Model file for the job. Use its own axes, mm. A direction names the side the tool comes from. Coordinates: 2 decimals unless noted, no trailing zeros. Write each loop counter-clockwise with the first axis right and the second up, starting at its lowest first coordinate (ties: lowest second). Pieces come first, ordered by that corner, then holes. Notation, with made-up numbers: (-11, 0) - (8, 0) arc R25 cw to (8, 27) - close; hole circle Ø10 at (73, 14). An arc over 180 degrees is marked (long way). Put each result on its own line as item: value. Start each with the question number.
1. Saw through at B-B, the plane z = 68. Write the cut outline in (x, y).
2. Pull direction Z, two halves, no side cores. Call faces 3 (the face through (138.4, -12.52, 41.08)), 4 (the face through (7, -25.4, 37)), 5 (the face through (-76.09, -12.52, 7.42)), 6 (the face through (24.914, -13, -1)): released by +Z, released by -Z, zero draft, split by the parting line, or undercut.
3. Saw through at A-A, the plane x = -2.5. Write the cut outline in (y, z).
4. Which spindle directions (+Z, -Z, +X, -X, +Y, -Y) get a long thin tool onto all of the face, cutting with end or side? Do faces 1 (the face through (0.354, -12.522, 20.673)), 2 (the face through (75.2, -12.522, -8.387)). Say none if no direction does.
5. Drill centre lines: L1, parallel to X at y = -13.25, z = 58.5; L2, parallel to X at y = -10.25, z = 65; L3, parallel to X at y = -11, z = 56. Where is each one in solid material? Low to high. Write a range as from..to.
6. Drop flat-ended pins along their axis: P1, Ø4, axis at x = 65, y = -3.5, coming from the +Z side; P2, Ø10, axis at x = -74.5, y = -20.5, coming from the +Z side; P3, Ø4, axis at x = -22.5, y = -6.5, coming from the -Z side. Give the stop position or say it passes through.
7. Saw through at C-C, the plane y = -9.25. Write the cut outline in (x, z), plus the area to 3 significant figures.
8. Saw through at D-D, the plane x = -50.5. Write the cut outline in (y, z), plus the area to 3 significant figures.
```python
from build123d import *

# Parameters (mm, degrees)
F0_R     = 13.5638253362
F1_DEPTH = 25.4
F2_DEPTH = 41.656
F3_DEPTH = 26.162


with BuildPart() as f1:
    # F0 (on Front) → F1 (new body)
    with BuildSketch(Plane.XZ):
        with BuildLine():
            ThreePointArc((42.2479079596, 0), (36.1330221503, -21.892702831), (19.5584797538, -37.4479852152))
            Line((19.5584797538, -37.4479852152), (132.4212052928, 21.4983992089))
            ThreePointArc((132.4212052928, 21.4983992089), (100.6472035915, 41.7404632116), (123.3718206821, 71.7890924196))
            Line((123.3718206821, 71.7890924196), (-99.4221599354, 82.6346792182))
            ThreePointArc((-99.4221599354, 82.6346792182), (-91.712695746, 74.4613506675), (-88.9104630026, 63.580788672))
            ThreePointArc((-88.9104630026, 63.580788672), (-98.9866948233, 44.8085061449), (-120.2003748087, 42.8314324344))
            Line((-120.2003748087, 42.8314324344), (-30.734153315, -28.9878862108))
            ThreePointArc((-30.734153315, -28.9878862108), (-15.5953846777, 39.2641019726), (42.2479079596, 0))
        make_face()
        with BuildLine():
            Line((-30.734153315, -28.9878862108), (-21.6561091574, -36.2753175468))
            ThreePointArc((-21.6561091574, -36.2753175468), (-1.201582142, -42.2308172703), (19.5584797538, -37.4479852152))
            ThreePointArc((19.5584797538, -37.4479852152), (36.1330221503, -21.892702831), (42.2479079596, 0))
            ThreePointArc((42.2479079596, 0), (-15.5953846777, 39.2641019726), (-30.734153315, -28.9878862108))
        make_face()
        with BuildLine():
            ThreePointArc((-19.4369487029, 7.0494087413), (0, 20.6758104674), (19.4369487029, 7.0494087413))
            Line((19.4369487029, 7.0494087413), (24.9135568738, 7.0494087413))
            Line((24.9135568738, 7.0494087413), (24.9135568738, -8.5022896528))
            Line((24.9135568738, -8.5022896528), (18.8467559315, -8.5022896528))
            ThreePointArc((18.8467559315, -8.5022896528), (0, -20.6758104674), (-18.8467559315, -8.5022896528))
            Line((-18.8467559315, -8.5022896528), (-24.5691239834, -8.5022896528))
            Line((-24.5691239834, -8.5022896528), (-24.5691239834, 7.0494087413))
            Line((-24.5691239834, 7.0494087413), (-19.4369487029, 7.0494087413))
        make_face(mode=Mode.SUBTRACT)
        with BuildLine():
            ThreePointArc((123.3718206821, 71.7890924196), (100.6472035915, 41.7404632116), (132.4212052928, 21.4983992089))
            ThreePointArc((132.4212052928, 21.4983992089), (146.1814974644, 30.6406644058), (151.5054987025, 46.2797712983))
            ThreePointArc((151.5054987025, 46.2797712983), (143.0908574497, 65.2681184027), (123.3718206821, 71.7890924196))
        make_face()
        with Locations((125.873775364, 46.2797712983)):
            Circle(F0_R, mode=Mode.SUBTRACT)
        with BuildLine():
            Line((-129.7982639681, 50.536171143), (-120.2003748087, 42.8314324344))
            ThreePointArc((-120.2003748087, 42.8314324344), (-98.9866948233, 44.8085061449), (-88.9104630026, 63.580788672))
            ThreePointArc((-88.9104630026, 63.580788672), (-91.712695746, 74.4613506675), (-99.4221599354, 82.6346792182))
            ThreePointArc((-99.4221599354, 82.6346792182), (-127.7954989327, 79.063190443), (-129.7982639681, 50.536171143))
        make_face()
        with Locations((-111.4352047443, 63.580788672)):
            Circle(F0_R, mode=Mode.SUBTRACT)
        with BuildLine():
            ThreePointArc((18.8467559315, -8.5022896528), (20.2133754238, -4.3484011382), (20.6758104674, 0))
            ThreePointArc((20.6758104674, 0), (20.3637399061, 3.5787198156), (19.4369487029, 7.0494087413))
            Line((19.4369487029, 7.0494087413), (-19.4369487029, 7.0494087413))
            ThreePointArc((-19.4369487029, 7.0494087413), (-20.6609375603, -0.784090309), (-18.8467559315, -8.5022896528))
            Line((-18.8467559315, -8.5022896528), (18.8467559315, -8.5022896528))
        make_face()
        with Locations((-111.4352047443, 63.580788672)):
            Circle(F0_R)
        with Locations((125.873775364, 46.2797712983)):
            Circle(F0_R)
        with BuildLine():
            Line((-19.4369487029, 7.0494087413), (19.4369487029, 7.0494087413))
            ThreePointArc((19.4369487029, 7.0494087413), (0, 20.6758104674), (-19.4369487029, 7.0494087413))
        make_face()
        with BuildLine():
            ThreePointArc((-18.8467559315, -8.5022896528), (0, -20.6758104674), (18.8467559315, -8.5022896528))
            Line((18.8467559315, -8.5022896528), (-18.8467559315, -8.5022896528))
        make_face()
        with BuildLine():
            ThreePointArc((19.4369487029, 7.0494087413), (20.3637399061, 3.5787198156), (20.6758104674, 0))
            ThreePointArc((20.6758104674, 0), (20.2133754238, -4.3484011382), (18.8467559315, -8.5022896528))
            Line((18.8467559315, -8.5022896528), (24.9135568738, -8.5022896528))
            Line((24.9135568738, -8.5022896528), (24.9135568738, 7.0494087413))
            Line((24.9135568738, 7.0494087413), (19.4369487029, 7.0494087413))
        make_face()
        with BuildLine():
            ThreePointArc((-18.8467559315, -8.5022896528), (-20.6609375603, -0.784090309), (-19.4369487029, 7.0494087413))
            Line((-19.4369487029, 7.0494087413), (-24.5691239834, 7.0494087413))
            Line((-24.5691239834, 7.0494087413), (-24.5691239834, -8.5022896528))
            Line((-24.5691239834, -8.5022896528), (-18.8467559315, -8.5022896528))
        make_face()
        with BuildLine():
            ThreePointArc((-129.7982639681, 50.536171143), (-125.5357705386, 46.0155378963), (-120.2003748087, 42.8314324344))
            Line((-120.2003748087, 42.8314324344), (-129.7982639681, 50.536171143))
        make_face()
        with BuildLine():
            ThreePointArc((-30.734153315, -28.9878862108), (-26.4473356759, -32.9457760966), (-21.6561091574, -36.2753175468))
            Line((-21.6561091574, -36.2753175468), (-30.734153315, -28.9878862108))
        make_face()
    extrude(amount=F1_DEPTH)

    # F0 (on Front) → F2 (cut)
    with BuildSketch(Plane.XZ):
        with BuildLine():
            ThreePointArc((-18.8467559315, -8.5022896528), (0, -20.6758104674), (18.8467559315, -8.5022896528))
            Line((18.8467559315, -8.5022896528), (-18.8467559315, -8.5022896528))
        make_face()
        with BuildLine():
            Line((-19.4369487029, 7.0494087413), (19.4369487029, 7.0494087413))
            ThreePointArc((19.4369487029, 7.0494087413), (0, 20.6758104674), (-19.4369487029, 7.0494087413))
        make_face()
        with BuildLine():
            ThreePointArc((-18.8467559315, -8.5022896528), (-20.6609375603, -0.784090309), (-19.4369487029, 7.0494087413))
            Line((-19.4369487029, 7.0494087413), (-24.5691239834, 7.0494087413))
            Line((-24.5691239834, 7.0494087413), (-24.5691239834, -8.5022896528))
            Line((-24.5691239834, -8.5022896528), (-18.8467559315, -8.5022896528))
        make_face()
        with BuildLine():
            ThreePointArc((19.4369487029, 7.0494087413), (20.3637399061, 3.5787198156), (20.6758104674, 0))
            ThreePointArc((20.6758104674, 0), (20.2133754238, -4.3484011382), (18.8467559315, -8.5022896528))
            Line((18.8467559315, -8.5022896528), (24.9135568738, -8.5022896528))
            Line((24.9135568738, -8.5022896528), (24.9135568738, 7.0494087413))
            Line((24.9135568738, 7.0494087413), (19.4369487029, 7.0494087413))
        make_face()
        with BuildLine():
            ThreePointArc((18.8467559315, -8.5022896528), (20.2133754238, -4.3484011382), (20.6758104674, 0))
            ThreePointArc((20.6758104674, 0), (20.3637399061, 3.5787198156), (19.4369487029, 7.0494087413))
            Line((19.4369487029, 7.0494087413), (-19.4369487029, 7.0494087413))
            ThreePointArc((-19.4369487029, 7.0494087413), (-20.6609375603, -0.784090309), (-18.8467559315, -8.5022896528))
            Line((-18.8467559315, -8.5022896528), (18.8467559315, -8.5022896528))
        make_face()
    extrude(amount=F2_DEPTH, mode=Mode.SUBTRACT)

    # F0 (on Front) → F3 (cut)
    with BuildSketch(Plane.XZ):
        with Locations((-111.4352047443, 63.580788672)):
            Circle(F0_R)
        with Locations((125.873775364, 46.2797712983)):
            Circle(F0_R)
    extrude(amount=F3_DEPTH, mode=Mode.SUBTRACT)


solid = f1.part
```
Final values:
1. outline: (-133.52, -25.4) - (-124.26, -25.4) - (-124.26, 0) - (-133.52, 0) - close; (-98.61, -25.4) - (139.48, -25.4) - (139.48, 0) - (-98.61, 0) - close
2. face 3: undercut
2. face 4: zero draft
2. face 5: released by -Z
2. face 6: undercut
3. outline: (-25.4, -42.17) - (0, -42.17) - (0, -20.52) - (-25.4, -20.52) - close; (-25.4, 20.52) - (0, 20.52) - (0, 77.92) - (-25.4, 77.92) - close
4. face 1: +Y, -Y
4. face 2: -Z, +X, +Y, -Y
5. L1: x = -133.38..-124.01, -98.86..119.99, 131.76..148.4
5. L2: x = -133.92..-124.92, -97.95..143.38
5. L3: x = -132.65..-122.68, -100.19..116.41, 135.33..149.59
6. P1: stops at z = 74.73
6. P2: stops at z = 81.66
6. P3: stops at z = -36.94
7. outline: (-120.2, 42.83) - (-30.73, -28.99) arc R42.25 ccw to (19.56, -37.45) - (132.42, 21.5) arc R25.63 ccw to (123.37, 71.79) - (-99.42, 82.63) arc R22.52 ccw (long way) to start; hole circle Ø27.13 at (-111.44, 63.58); hole (-24.57, -8.5) - (-18.85, -8.5) arc R20.68 ccw to (18.85, -8.5) - (24.91, -8.5) - (24.91, 7.05) - (19.44, 7.05) arc R20.68 ccw to (-19.44, 7.05) - (-24.57, 7.05) - close; hole circle Ø27.13 at (125.87, 46.28)
7. area: 20,300 mm²
8. outline: (-25.4, -13.12) - (0, -13.12) - (0, 80.25) - (-25.4, 80.25) - close
8. area: 2,370 mm²
